Could you check a few things on this model? Use its own coordinates, in mm. Give positions to 0.01 mm unless a question says otherwise; leave off trailing zeros. Loops run counter-clockwise (first coordinate to the right, second up) from the corner with the lowest first, then second, coordinate; pieces in that order, holes last. Notation, with made-up numbers: M 13,71 L 68,71 A35 ccw 68,108 Z; hole C 14.5,78.25 d3. An arc over 180 degrees is marked long. Return JSON: item names as keys, results as strings. Group by question number.
1. Please list where these lines run through material, in increasing order: line 1 (X direction, y = 82.5, z = 2.6); line 2 (Y direction, x = 182, z = 2.35); line 3 (X direction, y = 36, z = 4).
2. If we section it at A-A (y = 35): Write out the boundary of the cut face in (x, z).
3. If we section it at C-C (z = 3.5): State how many separate pieces and enclosed holes the cut face has, plus the area to 3 significant figures.
4. If we section it at B-B (x = 23.5): Write out the boundary of the cut face in (y, z), plus the area to 3 significant figures.
5. For pin 1 (2.5 mm diameter, centred on y = 82.5, z = 3, fed in from +X); pin 2 (2.5 mm diameter, centred on y = 83.5, z = 2, fed in from -X); pin 3 (2 mm diameter, centred on x = 50, z = 2, fed in from -Y), each with a flat end and sliding along its axis, tell me the tip position at first contact or that it passes through.
6. If we section it at D-D (x = 95.25): Write out the boundary of the cut face in (y, z).
```python
from build123d import *

# Parameters (mm, degrees)
BOSS_EXTRUDE1_DEPTH = 5.08
CUT_EXTRUDE2_DEPTH  = 219.330036922
CUT_EXTRUDE4_DEPTH  = 219.330036922
CUT_EXTRUDE5_DEPTH  = 219.330036922
CUT_EXTRUDE6_DEPTH  = 219.330036922


with BuildPart() as part:
    # Sketch1 → Boss-Extrude1 (new body)
    with BuildSketch(Plane.XY):
        Polygon((198.966666667, 76.2), (198.966666667, 67.733333333), (190.5, 67.733333333), (190.5, 8.466666667), (198.966666667, 8.466666667), (198.966666667, 0), (190.5, 0), (190.5, -13.546666667), (177.8, -13.546666667), (177.8, 0), (12.7, 0), (12.7, -13.546666667), (0, -13.546666667), (0, 0), (-8.466666667, 0), (-8.466666667, 8.466666667), (0, 8.466666667), (0, 67.733333333), (-8.466666667, 67.733333333), (-8.466666667, 76.2), (0, 76.2), (0, 89.746666667), (12.7, 89.746666667), (12.7, 76.2), (177.8, 76.2), (177.8, 89.746666667), (190.5, 89.746666667), (190.5, 76.2), align=None)
    extrude(amount=BOSS_EXTRUDE1_DEPTH)

    # Sketch2 → Cut-Extrude2 (cut, through all)
    with BuildSketch(Plane.XY.offset(5.08)):
        with BuildLine():
            Line((95.25, 0), (115.316, 0))
            Line((115.316, 0), (115.316, 27.686))
            ThreePointArc((115.316, 27.686), (95.25, 47.752), (75.184, 27.686))
            Line((75.184, 27.686), (75.184, 0))
            Line((75.184, 0), (95.25, 0))
        make_face()
    extrude(amount=-CUT_EXTRUDE2_DEPTH, mode=Mode.SUBTRACT)

    # Sketch3 → Cut-Extrude4 (cut, through all)
    with BuildSketch(Plane.XY.offset(5.08)):
        Polygon((6.35, 81.28), (10.033, 81.28), (10.033, 86.36), (2.667, 86.36), (2.667, 81.28), align=None)
        Polygon((184.15, 81.28), (187.833, 81.28), (187.833, 86.36), (180.467, 86.36), (180.467, 81.28), align=None)
        Polygon((184.15, -5.08), (187.833, -5.08), (187.833, -10.16), (180.467, -10.16), (180.467, -5.08), align=None)
        Polygon((6.35, -5.08), (10.033, -5.08), (10.033, -10.16), (2.667, -10.16), (2.667, -5.08), align=None)
    extrude(amount=-CUT_EXTRUDE4_DEPTH, mode=Mode.SUBTRACT)

    # Sketch4 → Cut-Extrude5 (cut, through all)
    with BuildSketch(Plane.XY.offset(5.08)):
        Polygon((136.525, 5.08), (139.065, 5.08), (139.065, 12.7), (133.985, 12.7), (133.985, 5.08), align=None)
        Polygon((53.975, 5.08), (56.515, 5.08), (56.515, 12.7), (51.435, 12.7), (51.435, 5.08), align=None)
    extrude(amount=-CUT_EXTRUDE5_DEPTH, mode=Mode.SUBTRACT)

    # Sketch5 → Cut-Extrude6 (cut, through all)
    with BuildSketch(Plane.XY.offset(5.08)):
        Polygon((12.7, 67.733333333), (12.7, 8.466666667), (71.966666667, 67.733333333), align=None)
    cut_extrude6 = extrude(amount=-CUT_EXTRUDE6_DEPTH, mode=Mode.SUBTRACT)

    # Mirror1: Cut-Extrude6 across plane
    add(cut_extrude6.mirror(Plane(origin=(95.25, 0, 0), x_dir=(0, 0, 1), z_dir=(1, 0, 0))), mode=Mode.SUBTRACT)


solid = part.part
```
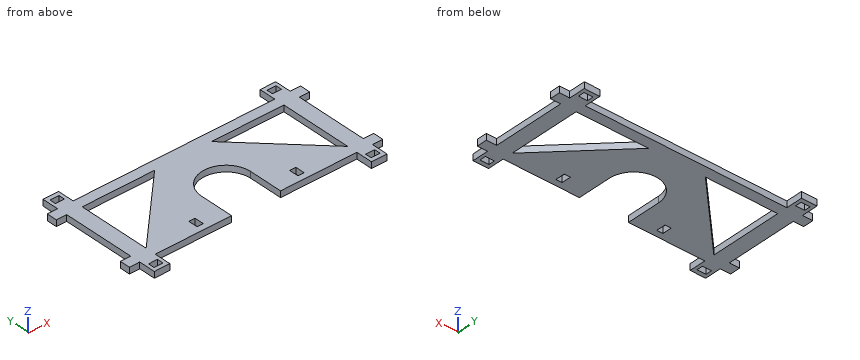
Answer:
{
 "1": {"line 1": "x = 0 to 2.67, 10.03 to 12.7, 177.8 to 180.47, 187.83 to 190.5", "line 2": "y = -13.55 to -10.16, -5.08 to 81.28, 86.36 to 89.75", "line 3": "x = 0 to 12.7, 40.23 to 76.99, 113.51 to 150.27, 177.8 to 190.5"},
 "2": {"outline": "M 0,0 L 12.7,0 L 12.7,5.08 L 0,5.08 Z; M 39.23,0 L 76.56,0 L 76.56,5.08 L 39.23,5.08 Z; M 113.94,0 L 151.27,0 L 151.27,5.08 L 113.94,5.08 Z; M 177.8,0 L 190.5,0 L 190.5,5.08 L 177.8,5.08 Z"},
 "3": {"separate pieces": "1", "enclosed holes": "8", "area": "10,000 mm²"},
 "4": {"outline": "M 0,0 L 19.27,0 L 19.27,5.08 L 0,5.08 Z; M 67.73,0 L 76.2,0 L 76.2,5.08 L 67.73,5.08 Z", "area": "141 mm²"},
 "5": {"pin 1": "stops at x = 190.5", "pin 2": "stops at x = 0", "pin 3": "stops at y = 0"},
 "6": {"outline": "M 47.75,0 L 76.2,0 L 76.2,5.08 L 47.75,5.08 Z"}
}
